Geometry: final body of the model. Coordinates: model frame, mm. A direction names the side the tool comes from. Round coordinates to 2 decimals unless told otherwise and drop trailing zeros. Loops run counter-clockwise (first coordinate to the right, second up) from the corner with the lowest first, then second, coordinate; pieces in that order, holes last. Notation, with made-up numbers: M -16.75,50 L 1.25,50 A12 cw 1.25,65 Z; hole C -29.5,12 d10. An arc over 180 degrees is marked long. Answer as a JSON object with one key per item and string values.
```python
from build123d import *

# Parameters (mm, degrees)
F0_W     = 508
F0_H     = 508
F0_W_2   = 88.9
F0_H_2   = 88.9
F1_DEPTH = 25.4
F2_DEPTH = 101.6
F3_DEPTH = 482.6
F4_R     = 88.89999
F5_R     = 25.4


# Not quite as in the source:
# - a fillet or chamfer is up to 0.001 mm smaller than in the source, because OpenCascade refuses the exact size


with BuildPart() as f1:
    # F0 (on Top) → F1 (new body)
    with BuildSketch(Plane.XY):
        Rectangle(F0_W, F0_H)
        Polygon((139.7, 228.6), (228.6, 228.6), (228.6, 139.7), (228.6, -139.7), (228.6, -228.6), (139.7, -228.6), (-139.7, -228.6), (-228.6, -228.6), (-228.6, -139.7), (-228.6, 139.7), (-228.6, 228.6), (-139.7, 228.6), align=None, mode=Mode.SUBTRACT)
        with Locations((-184.15, -184.15)):
            Rectangle(F0_W_2, F0_H_2)
        with Locations((184.15, -184.15)):
            Rectangle(F0_W_2, F0_H_2)
        with Locations((184.15, 184.15)):
            Rectangle(F0_W_2, F0_H_2)
        with Locations((-184.15, 184.15)):
            Rectangle(F0_W_2, F0_H_2)
        Polygon((139.7, 139.7), (139.7, 228.6), (-139.7, 228.6), (-139.7, 139.7), (-228.6, 139.7), (-228.6, -139.7), (-139.7, -139.7), (-139.7, -228.6), (139.7, -228.6), (139.7, -139.7), (228.6, -139.7), (228.6, 139.7), align=None)
    extrude(amount=-F1_DEPTH)

    # F0 (on Top) → F2 (join)
    with BuildSketch(Plane.XY):
        with Locations((-184.15, 184.15)):
            Rectangle(F0_W_2, F0_H_2)
        Polygon((139.7, 139.7), (139.7, 228.6), (-139.7, 228.6), (-139.7, 139.7), (-228.6, 139.7), (-228.6, -139.7), (-139.7, -139.7), (-139.7, -228.6), (139.7, -228.6), (139.7, -139.7), (228.6, -139.7), (228.6, 139.7), align=None)
        with Locations((184.15, 184.15)):
            Rectangle(F0_W_2, F0_H_2)
        with Locations((184.15, -184.15)):
            Rectangle(F0_W_2, F0_H_2)
        with Locations((-184.15, -184.15)):
            Rectangle(F0_W_2, F0_H_2)
    extrude(amount=-F2_DEPTH)

    # F0 (on Top) → F3 (join)
    with BuildSketch(Plane.XY):
        with Locations((-184.15, 184.15)):
            Rectangle(F0_W_2, F0_H_2)
        with Locations((-184.15, -184.15)):
            Rectangle(F0_W_2, F0_H_2)
        with Locations((184.15, 184.15)):
            Rectangle(F0_W_2, F0_H_2)
        with Locations((184.15, -184.15)):
            Rectangle(F0_W_2, F0_H_2)
    extrude(amount=-F3_DEPTH)

    # F4 (radius 88.9 in the source; OpenCascade refuses exactly that, so slightly less here)
    f4_edges = [f1.edges().sort_by_distance(p)[0] for p in [
        (-228.6, -228.6, -254),
        (228.6, -228.6, -254),
        (228.6, 228.6, -254),
        (-228.6, 228.6, -254),
    ]]
    fillet(f4_edges, radius=F4_R)

    # F5
    f5_edges = [f1.edges().sort_by_distance(p)[0] for p in [
        (254, -254, -12.7),
        (254, 254, -12.7),
        (-254, 254, -12.7),
        (-254, -254, -12.7),
    ]]
    fillet(f5_edges, radius=F5_R)


solid = f1.part
```
1) Cut plane A-A on z = -326. Count the separate pieces of the cut face and the enclosed holes in it, and give its area (3 significant figures).
Geometry results:
{"separate pieces": "4", "enclosed holes": "0", "area": "24,800 mm2"}
2) Pull-direction query (X, two-part tool) for faces 5 (the face through (-185, 139.7, -289)), 6 (the face through (139.7, 184, -289)), 7 (the face through (254, -3, -13)), 8 (the face through (-246.76, -246.36, -12.88)); classes: +X half, -X half, draft (parallel to the pull), parting line (faces both ways), or undercut.
Geometry results:
{"face 5": "draft", "face 6": "undercut", "face 7": "+X half", "face 8": "-X half"}
3) Line query: probe 1 along Z at (x, y) = (180.5, -60); probe 2 along X at (y, z) = (141, -307.5); probe 3 along X at (y, z) = (-21, -85). Output: solid intervals per line, ascending.
Geometry results:
{"probe 1": "-101.6 to 0", "probe 2": "-228.59 to -139.7, 139.7 to 228.59", "probe 3": "-228.6 to 228.6"}
4) Cut plane B-B on y = -80. Return the cut outline in (x, z).
Geometry results:
{"outline": "M -254,-25.4 L -228.6,-25.4 L -228.6,-101.6 L 228.6,-101.6 L 228.6,-25.4 L 254,-25.4 L 254,0 L -254,0 Z"}
5) Set-up query: faces 1 (the face through (203.249, 201.867, -250.8)), 2 (the face through (-185, -139.7, -289)), 3 (the face through (1, 228.6, -67)), 4 (the face through (139.7, -185, -289)). Return all of +Z, -Z, +X, -X, +Y, -Y with unobstructed straight access to the full face (end or side cutting, diameter ignored); none if empty.
Geometry results:
{"face 1": "-Z, +X, +Y", "face 2": "-Z, +X, -X", "face 3": "-Z, +X, -X, +Y", "face 4": "-Z, +Y, -Y"}
6) Cut plane D-D on x = -209.5. Return the cut outline in (y, z).
Geometry results:
{"outline": "M -254,-25.4 L -194.76,-25.4 L -194.76,-482.6 L -139.7,-482.6 L -139.7,-101.6 L 139.7,-101.6 L 139.7,-482.6 L 194.76,-482.6 L 194.76,-25.4 L 254,-25.4 L 254,0 L -254,0 Z"}
7) First-contact query: pin 1 (12 mm diameter, centred on x = -59, y = -71, fed in from +Z); pin 2 (1 mm diameter, centred on x = -95, y = 140, fed in from -Z). Flat tips, straight axial feed; report the tip coordinate or a pass-through.
Geometry results:
{"pin 1": "z = 0", "pin 2": "z = -101.6"}
